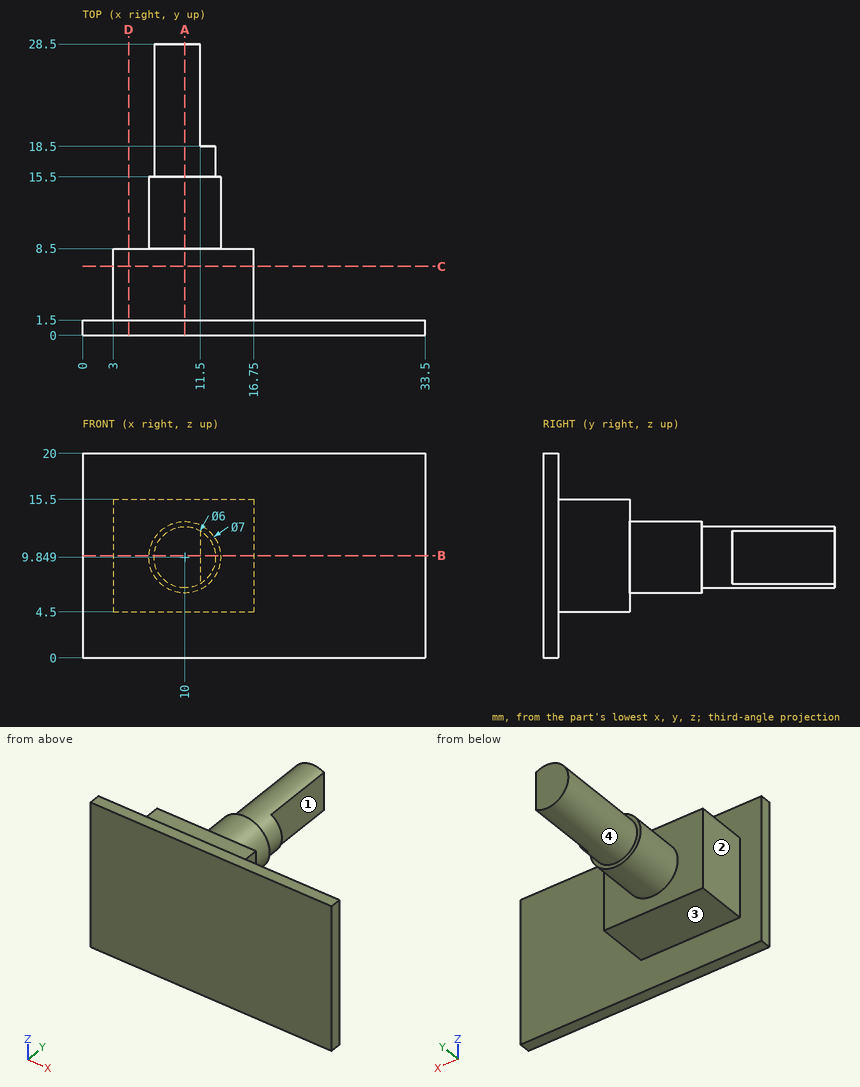
The drawing under review shows one solid part. Ordinate dimensions are in mm from its lowest x, y, z. A direction names the side the tool comes from. Give positions to 0.01 mm unless a question says otherwise; leave off trailing zeros. Order: outer loops, then holes, each group sorted by start corner. A loop starts at its lowest first (then second) coordinate and runs counter-clockwise, first axis right, second up. Notation, with made-up numbers: M 47.25,5 L 78.25,5 A30 ccw 78.25,37 Z; hole C 89.25,10.5 d11. An arc over 180 degrees is marked long. One line per question, with ' | ' between items. Start each with the question number.
Q1. We need section B-B (z = 10). Write out the cut boundary in (x, y).
Q2. For pin 1 Ø6 at (y, z) = (5.5, 17.5) entering from -X; pin 2 Ø10 at (x, z) = (28.5, 5.5) entering from +Y; pin 3 Ø0.5 at (x, z) = (12.5, 9) entering from +Y; pin 4 Ø5 at (y, z) = (25, 17) entering from +X, all flat-tipped, find the tip position at first contact; note any pin that passes through.
Q3. We need section A-A (x = 10). Write out the cut boundary in (y, z), plus the area to 3 significant figures.
Q4. We need section C-C (y = 6.75). Write out the cut boundary in (x, z).
Q5. For L1, parallel to Z at x = 9, y = 6.25; L2, parallel to Y at x = 9, z = 3.75; L3, parallel to X at y = 18.75, z = 8.5, list the stretches that pass through material, from the lowest coordinate up. Write a range as [from, to].
Q6. Machinability: for the marked faces 1, 2, 3 and 4, which of the approach directions +Z, -Z, +X, -X, +Y, -Y give a long, thin tool a straight path to every point of the face, cutting with its end or side? Answer none if there is none.
Q7. We need section D-D (x = 4.5). Write out the cut boundary in (y, z).
Returned:
1) outline: M 0,0 L 33.5,0 L 33.5,1.5 L 16.75,1.5 L 16.75,8.5 L 13.5,8.5 L 13.5,15.5 L 13,15.5 L 13,18.5 L 11.5,18.5 L 11.5,28.5 L 7,28.5 L 7,15.5 L 6.5,15.5 L 6.5,8.5 L 3,8.5 L 3,1.5 L 0,1.5 Z
2) pin 1: x = 3 | pin 2: y = 1.5 | pin 3: y = 18.5 | pin 4: through
3) outline: M 0,0 L 1.5,0 L 1.5,4.5 L 8.5,4.5 L 8.5,6.35 L 15.5,6.35 L 15.5,6.85 L 28.5,6.85 L 28.5,12.85 L 15.5,12.85 L 15.5,13.35 L 8.5,13.35 L 8.5,15.5 L 1.5,15.5 L 1.5,20 L 0,20 Z | area: 234 mm2
4) outline: M 3,4.5 L 16.75,4.5 L 16.75,15.5 L 3,15.5 Z
5) L1: [4.5, 15.5] | L2: [0, 1.5] | L3: [7.32, 11.5]
6) face 1: +Z, -Z, +X, +Y | face 2: +Z, -Z, -X, +Y | face 3: -Z, +X, -X, +Y | face 4: +Y
7) outline: M 0,0 L 1.5,0 L 1.5,4.5 L 8.5,4.5 L 8.5,15.5 L 1.5,15.5 L 1.5,20 L 0,20 Z
